```python
from build123d import *

# Parameters (mm, degrees)
F0_R     = 19.248811
F2_DEPTH = 5
F1_R     = 10
F3_DEPTH = 2
F1_R_2   = 16.619504
F1_R_3   = 13.327502
F4_DEPTH = 25
F5_DEPTH = 2


with BuildPart() as f2:
    # F0 (on Front) → F2 (new body)
    with BuildSketch(Plane.XZ):
        Circle(F0_R)
    extrude(amount=F2_DEPTH)

    # F1 (on Front) → F3 (cut)
    with BuildSketch(Plane.XZ):
        Circle(F1_R)
    extrude(amount=F3_DEPTH, mode=Mode.SUBTRACT)

    # F1 (on Front) → F4 (join)
    with BuildSketch(Plane.XZ):
        Circle(F1_R_2)
        Circle(F1_R_3, mode=Mode.SUBTRACT)
    extrude(amount=F4_DEPTH)

    # F1 (on Front) → F5 (cut)
    with BuildSketch(Plane.XZ):
        Circle(F1_R_2)
        Circle(F1_R_3, mode=Mode.SUBTRACT)
    extrude(amount=F5_DEPTH, mode=Mode.SUBTRACT)


solid = f2.part
```
Verification items for the finished model (mm, model axes). A direction names the side the tool comes from. Round coordinates to 2 decimals unless told otherwise and drop trailing zeros. Loops run counter-clockwise (first coordinate to the right, second up) from the corner with the lowest first, then second, coordinate; pieces in that order, holes last. Notation, with made-up numbers: (-27, 37) -> (20, 37) arc R13 cw to (20, 55) -> close; hole circle Ø11 at (-6.5, 1.5). An arc over 180 degrees is marked (long way). Answer as a JSON object with one key per item and string values.
Q1. Section check D-D (x = -16). Record the boundary of the cut face in (y, z), then the cut area to 3 significant figures.
Data:
{"outline": "(-25, -4.5) -> (-5, -4.5) -> (-5, -10.7) -> (0, -10.7) -> (0, -4.5) -> (-2, -4.5) -> (-2, 4.5) -> (0, 4.5) -> (0, 10.7) -> (-5, 10.7) -> (-5, 4.5) -> (-25, 4.5) -> close", "area": "269 mm2"}
Q2. Section check B-B (z = 0). Record the boundary of the cut face in (x, y).
Data:
{"outline": "(-19.25, -5) -> (-16.62, -5) -> (-16.62, -25) -> (-13.33, -25) -> (-13.33, -5) -> (13.33, -5) -> (13.33, -25) -> (16.62, -25) -> (16.62, -5) -> (19.25, -5) -> (19.25, 0) -> (16.62, 0) -> (16.62, -2) -> (13.33, -2) -> (13.33, 0) -> (10, 0) -> (10, -2) -> (-10, -2) -> (-10, 0) -> (-13.33, 0) -> (-13.33, -2) -> (-16.62, -2) -> (-16.62, 0) -> (-19.25, 0) -> close"}
Q3. Section check A-A (x = 0). Record the boundary of the cut face in (y, z).
Data:
{"outline": "(-25, -16.62) -> (-5, -16.62) -> (-5, -19.25) -> (0, -19.25) -> (0, -16.62) -> (-2, -16.62) -> (-2, -13.33) -> (0, -13.33) -> (0, -10) -> (-2, -10) -> (-2, 10) -> (0, 10) -> (0, 13.33) -> (-2, 13.33) -> (-2, 16.62) -> (0, 16.62) -> (0, 19.25) -> (-5, 19.25) -> (-5, 16.62) -> (-25, 16.62) -> (-25, 13.33) -> (-5, 13.33) -> (-5, -13.33) -> (-25, -13.33) -> close"}
Q4. Access from +Z, -Z, +X, -X, +Y, -Y to the whole of each face (thin tool, end or side, straight path). Record for faces 1 (the flat face through (0, -25, 14)), 2 (the flat face through (0, -5, 0)), 3 (the cylindrical face through (12.712, -0.986, 4.003)).
Data:
{"face 1": "+Z, -Z, +X, -X, -Y", "face 2": "-Y", "face 3": "+Y"}
Q5. Draft check along Z on faces 4 (the cylindrical face through (18.36, -2.46, 5.78)), 5 (the flat face through (2, 0, 10)), 6 (the cylindrical face through (12.712, -14.86, 4.003)). Enter one of: pulls with the +Z half, pulls with the -Z half, needs draft (parallel to the pull), parting line crosses it, or undercut.
Data:
{"face 4": "parting line crosses it", "face 5": "needs draft", "face 6": "undercut"}
Q6. Scan lines: line 1 (Z direction, x = 0, y = -0.5); line 2 (X direction, y = -10.5, z = 0). Record each from-to range of solid material in increasing order. Write a range as from..to.
Data:
{"line 1": "z = -19.25..-16.62, -13.33..-10, 10..13.33, 16.62..19.25", "line 2": "x = -16.62..-13.33, 13.33..16.62"}
Q7. Section check C-C (y = -11.25). Record the boundary of the cut face in (x, z) (1 decimal), then the cut area to 3 significant figures.
Data:
{"outline": "circle Ø33.2 at (0, 0); hole circle Ø26.7 at (0, 0)", "area": "310 mm2"}
Q8. Go/stop test with flat-tipped pins: P1, Ø2, axis at x = -13, y = -19, coming from the +Z side; P2, Ø1, axis at x = -8.5, y = -4, coming from the -Z side; P3, Ø10, axis at x = 1, z = -4, coming from the +Y side. Record where each tip stops, or that it passes through.
Data:
{"P1": "stops at z = 11.5", "P2": "stops at z = -17.51", "P3": "stops at y = -2"}
